Geometry: final body of the model. Coordinates: model frame, mm. A direction names the side the tool comes from. Give positions to 0.01 mm unless a question says otherwise; leave off trailing zeros. Write each loop counter-clockwise with the first axis right and the second up, starting at its lowest first coordinate (ties: lowest second). Pieces come first, ordered by that corner, then holes. Notation, with made-up numbers: M 30,-6.75 L 47,-6.75 A28 ccw 47,20.25 Z; hole C -30.5,-29 d5. An arc over 180 degrees is marked long. Use a Markdown table: item, result. Add a question column.
1) Line query: line 1 (Z direction, x = 11.5, y = 1.5); line 2 (X direction, y = 9.25, z = 18.5); line 3 (Z direction, x = -28.5, y = 6.25). Output: solid intervals per line, ascending.
2) Pin query (flat end, axial travel): pin 1 (6 mm diameter, centred on y = 12.5, z = 9, fed in from -X); pin 2 (2.5 mm diameter, centred on x = 11.5, z = 30.67, fed in from +Y); pin 3 (8 mm diameter, centred on x = -22, y = 11.5, fed in from +Z). Return the tip coordinate at first contact, or that it passes through.
3) Section B-B on y = 1.5. Return the cut outline in (x, z) (3 decimals), then the cut area to 3 significant figures.
4) Draft query along Z for faces 4 (the flat face through (0, 3, 8)), 5 (the cylindrical face through (11.28, 1.52, 31.67)), 6 (the flat face through (-15.48, 11.38, 18.72)). Return one class per face: +Z half, -Z half, draft (parallel to the pull), parting line (faces both ways), or undercut.
5) Section C-C on z = 25. Return the cut outline in (x, y), then the cut area to 3 significant figures.
6) Section A-A on x = 8. Return the cut outline in (y, z).
7) Section D-D on y = 10.75. Return the cut outline in (x, z).
8) Set-up query: faces 1 (the flat face through (0, 12, 3)), 2 (the flat face through (21.6, 11.6, 3)), 3 (the flat face through (21, 3, 1)). Return all of +Z, -Z, +X, -X, +Y, -Y with unobstructed straight access to the full face (end or side cutting, diameter ignored); none if empty.
```python
from build123d import *

# Parameters (mm, degrees)
BOSS_EXTRUDE2_DEPTH = 17
RIB2_REACH          = 54.077
SKETCH5_WALL_W      = 141.50907159
SKETCH5_WALL_H      = 3
SKETCH6_R           = 2.5
BOSS_EXTRUDE3_DEPTH = 3
CUT_EXTRUDE1_DEPTH  = 3


with BuildPart() as part:
    # Sketch2 → Boss-Extrude2 (new, symmetric)
    with BuildSketch(Plane(origin=(0, 0, 0), x_dir=(0, 0, -1), z_dir=(1, 0, 0))):
        Polygon((0, 0), (0, 20), (-3, 20), (-3, 3), (-34, 3), (-34, 0), align=None)
    extrude(amount=BOSS_EXTRUDE2_DEPTH, both=True)

    # Sketch5 wall → Rib2 (add, up to next)
    with BuildSketch(Plane(origin=(17, 11.5, 18.5), x_dir=(0, 0.480832611207, -0.876812408671), z_dir=(0, 0.876812408671, 0.480832611207)), mode=Mode.PRIVATE) as rib2_sk1:
        with Locations((0, 1.5)):
            Rectangle(SKETCH5_WALL_W, SKETCH5_WALL_H)
    rib2_tool1 = extrude(rib2_sk1.sketch, amount=-RIB2_REACH, mode=Mode.PRIVATE) - part.part
    rib2 = rib2_tool1.solids().sort_by_distance((17, 11.5, 18.5))[0]
    add(rib2)

    # Sketch6 → Boss-Extrude3 (add)
    with BuildSketch(Plane.XY):
        with BuildLine():
            Line((17, 20), (24.5, 20))
            ThreePointArc((24.5, 20), (33, 11.5), (24.5, 3))
            Line((24.5, 3), (17, 3))
            Line((17, 3), (17, 20))
        make_face()
        with Locations((24.5, 11.5)):
            Circle(SKETCH6_R, mode=Mode.SUBTRACT)
    boss_extrude3 = extrude(amount=BOSS_EXTRUDE3_DEPTH)

    # Mirror1: Rib2, Boss-Extrude3 across plane
    add(rib2.mirror(Plane(origin=(0, 0, 0), x_dir=(0, 0, 1), z_dir=(1, 0, 0))))
    add(boss_extrude3.mirror(Plane(origin=(0, 0, 0), x_dir=(0, 0, 1), z_dir=(1, 0, 0))))

    # Sketch8 → Cut-Extrude1 (cut)
    with BuildSketch(Plane(origin=(0, 3, 0), x_dir=(1, 0, 0), z_dir=(0, 1, 0))):
        with BuildLine():
            ThreePointArc((11, -19.168010742), (0, -8.168010742), (-11, -19.168010742))
            ThreePointArc((-11, -19.168010742), (0, -30.168010742), (11, -19.168010742))
        make_face()
        with BuildLine():
            ThreePointArc((-10.475, -7.668010742), (-11.5, -6.643010742), (-12.525, -7.668010742))
            ThreePointArc((-12.525, -7.668010742), (-11.5, -8.693010742), (-10.475, -7.668010742))
        make_face()
        with BuildLine():
            ThreePointArc((-12.525, -30.668010742), (-11.5, -31.693010742), (-10.475, -30.668010742))
            ThreePointArc((-10.475, -30.668010742), (-11.5, -29.643010742), (-12.525, -30.668010742))
        make_face()
        with BuildLine():
            ThreePointArc((10.475, -7.668010742), (11.5, -8.693010742), (12.525, -7.668010742))
            ThreePointArc((12.525, -7.668010742), (11.5, -6.643010742), (10.475, -7.668010742))
        make_face()
        with BuildLine():
            ThreePointArc((10.475, -30.668010742), (11.5, -31.693010742), (12.525, -30.668010742))
            ThreePointArc((12.525, -30.668010742), (11.5, -29.643010742), (10.475, -30.668010742))
        make_face()
    extrude(amount=-CUT_EXTRUDE1_DEPTH, mode=Mode.SUBTRACT)


solid = part.part
```
Found:
| question | item | result |
|---|---|---|
| 1 | line 1 | 0 to 6.64, 8.69 to 29.64, 31.69 to 34 |
| 1 | line 2 | -17 to -14, 14 to 17 |
| 1 | line 3 | 0 to 3 |
| 2 | pin 1 | x = -17 |
| 2 | pin 2 | y = 3 |
| 2 | pin 3 | z = 3 |
| 3 | outline | M -17,0 L 17,0 L 17,34 L -17,34 Z; hole C -11.5,7.668 d2.05; hole C -11.5,30.668 d2.05; hole C 0,19.168 d22; hole C 11.5,7.668 d2.05; hole C 11.5,30.668 d2.05 |
| 3 | area | 763 mm² |
| 4 | face 4 | draft |
| 4 | face 5 | undercut |
| 4 | face 6 | +Z half |
| 5 | outline | M -17,0 L -9.33,0 L -9.33,3 L -14,3 L -14,7.94 L -17,7.94 Z; M 9.33,0 L 17,0 L 17,7.94 L 14,7.94 L 14,3 L 9.33,3 Z |
| 5 | area | 75.7 mm² |
| 6 | outline | M 0,0 L 20,0 L 20,3 L 3,3 L 3,11.62 L 0,11.62 Z; M 0,26.72 L 3,26.72 L 3,34 L 0,34 Z |
| 7 | outline | M -32.97,0 L -26.88,0 L -26.88,3 L -32.97,3 Z; M -22.12,0 L 22.12,0 L 22.12,3 L 17,3 L 17,19.87 L 14,19.87 L 14,3 L -14,3 L -14,19.87 L -17,19.87 L -17,3 L -22.12,3 Z; M 26.88,0 L 32.97,0 L 32.97,3 L 26.88,3 Z |
| 8 | face 1 | +Z, +Y |
| 8 | face 2 | +Z, +X, +Y, -Y |
| 8 | face 3 | +Z, -Z, +X, -Y |
